Geometry check sheet. Reference: the model listing, model coordinates, mm. Face numbers are marked on the shaded views. A direction names the side the tool comes from. Round coordinates to 2 decimals unless told otherwise and drop trailing zeros. Write each loop counter-clockwise with the first axis right and the second up, starting at its lowest first coordinate (ties: lowest second). Pieces come first, ordered by that corner, then holes. Notation, with made-up numbers: (-30.75, 58) -> (15.25, 58) arc R10 ccw to (15.25, 62) -> close; hole circle Ø9 at (30, 33). An arc over 180 degrees is marked (long way). One line per question, with ' | ' between items.
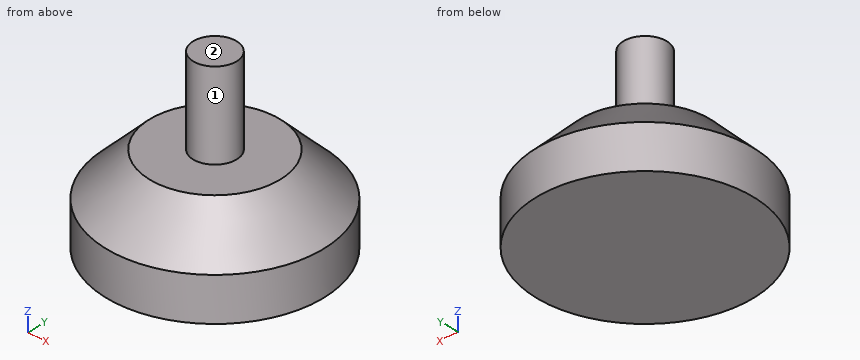
```python
from build123d import *

# Parameters (mm, degrees)
F0_R     = 31.75
F1_DEPTH = 25.4
F2_SIZE  = 12.7
F3_R     = 6.35
F4_DEPTH = 25.4


with BuildPart() as f1:
    # F0 (on Top) → F1 (new body)
    with BuildSketch(Plane.XY):
        Circle(F0_R)
    extrude(amount=F1_DEPTH)

    # F2
    f2_edges = [f1.edges().sort_by_distance(p)[0] for p in [
        (-31.75, 0, 25.4),
    ]]
    chamfer(f2_edges, length=F2_SIZE)

    # F3 (on face) → F4 (join)
    with BuildSketch(Plane.XY.offset(25.4)):
        Circle(F3_R)
    extrude(amount=F4_DEPTH)


solid = f1.part
```
(1) Sectioned sample at D-D on z = 44. Record the cut outline in (x, y), then the cut area to 3 significant figures.
Resolved:
outline: circle Ø12.7 at (0, 0) | area: 127 mm2
(2) Go/stop test with flat-tipped pins: pin 1 (6 mm diameter, centred on y = 7, z = 12, fed in from +X); pin 2 (1 mm diameter, centred on x = 11.5, z = 9, fed in from +Y); pin 3 (8 mm diameter, centred on x = -9.5, z = 43, fed in from -Y); pin 4 (4 mm diameter, centred on x = 4, y = 13.5, fed in from -Z). Record where each tip stops, or that it passes through.
Resolved:
pin 1: stops at x = 31.5 | pin 2: stops at y = 29.78 | pin 3: stops at y = -3.17 | pin 4: stops at z = 0
(3) Material ranges on line 1 (Z direction, x = -10, y = 1.5); line 2 (Z direction, x = -20.5, y = 15); line 3 (Y direction, x = 6, z = 21), recorded low to high.
Resolved:
line 1: z = 0 to 25.4 | line 2: z = 0 to 19.05 | line 3: y = -22.67 to 22.67
(4) Sectioned sample at C-C on z = 19. Record the cut outline in (x, y), then the cut area to 3 significant figures.
Resolved:
outline: circle Ø50.9 at (0, 0) | area: 2,030 mm2
(5) Access from +Z, -Z, +X, -X, +Y, -Y to the whole of each face (thin tool, end or side, straight path). Record for the marked faces 1 and 2.
Resolved:
face 1: +Z | face 2: +Z, +X, -X, +Y, -Y
(6) Sectioned sample at A-A on y = 0. Record the cut outline in (x, z).
Resolved:
outline: (-31.75, 0) -> (31.75, 0) -> (31.75, 12.7) -> (19.05, 25.4) -> (6.35, 25.4) -> (6.35, 50.8) -> (-6.35, 50.8) -> (-6.35, 25.4) -> (-19.05, 25.4) -> (-31.75, 12.7) -> close
